from build123d import *

# Parameters (mm, degrees)
SKETCH_R      = 19.5
PAD_DEPTH     = 10
PAD001_START  = 10
SKETCH002_R   = 20
PAD001_DEPTH  = 110
SKETCH003_R   = 18.5
POCKET_DEPTH  = 120.001
PAD003_START  = 118
SKETCH007_R   = 30
SKETCH007_R_2 = 20
PAD003_DEPTH  = 2


with BuildPart() as part:
    # Sketch → Pad (new body)
    with BuildSketch(Plane.XY):
        Circle(SKETCH_R)
    extrude(amount=PAD_DEPTH)

    # Sketch002 → Pad001 (join)
    with BuildSketch(Plane.XY.offset(PAD001_START)):
        Circle(SKETCH002_R)
    extrude(amount=PAD001_DEPTH)

    # Sketch003 → Pocket (cut, through all)
    with BuildSketch(Plane.XY):
        Circle(SKETCH003_R)
    extrude(amount=POCKET_DEPTH, mode=Mode.SUBTRACT)

    # Sketch007 → Pad003 (join)
    with BuildSketch(Plane.XY.offset(PAD003_START)):
        Circle(SKETCH007_R)
        Circle(SKETCH007_R_2, mode=Mode.SUBTRACT)
    extrude(amount=PAD003_DEPTH)


solid = part.part
The model under review builds one solid part; all positions refer to its coordinate system, in mm. A direction names the side the tool comes from. Round coordinates to 2 decimals unless told otherwise and drop trailing zeros. Order: outer loops, then holes, each group sorted by start corner. A loop starts at its lowest first (then second) coordinate and runs counter-clockwise, first axis right, second up. Notation, with made-up numbers: (-39, -28.75) -> (-4, -28.75) arc R11 cw to (-4, -22.75) -> close; hole circle Ø9 at (70, -23.75). An arc over 180 degrees is marked (long way). Write item = value, one per line. Start each with the question number.
Item 1: Clearance check with flat-ended pins moving along their axes: pin 1 Ø6 at (y, z) = (-0.5, 24.5) entering from +X; pin 2 Ø1 at (y, z) = (-4, 33.5) entering from +X; pin 3 Ø1 at (y, z) = (6, 43.5) entering from -X. State where each tip first meets the part, or that it passes through.
Item 2: For faces 1 (the face through (19.2, -4.4, 10)), 2 (the face through (17.24, -7.13, 0)), list the 3-axis set-ups (+Z, -Z, +X, -X, +Y, -Y) from which the entire face can be reached by the end or side of a thin tool; tool diameter is ignored.
Item 3: For line 1 along Y through (x, z) = (0, 66); line 2 along Z through (x, y) = (-19, 7.5); line 3 along Y through (x, z) = (15, 9), list the stretches that pass through material, from the lowest coordinate up.
Item 4: Consider section A-A on x = 0. Write out the cut boundary in (y, z).
Item 5: Consider section C-C on z = 107.5. Write out the cut boundary in (x, y).
Item 6: Consider section D-D on y = -22.5. Write out the cut boundary in (x, z).
Item 7: Mouldability with a two-part tool opening along X and no side actions: class faces 3 (the face through (-4.01, -18.06, 59.16)), 4 (the face through (6, -20, 118)), 5 (the face through (-2.539, 19.334, 4.93)) as released by +X, released by -X, zero draft, split by the parting line, or undercut.
Conclusion:
q1.pin_1 = 20
q1.pin_2 = 19.69
q1.pin_3 = -19.23
q2.face_1 = -Z
q2.face_2 = -Z, +X, -X, +Y, -Y
q3.line_1 = -20 to -18.5, 18.5 to 20
q3.line_2 = 118 to 120
q3.line_3 = -12.46 to -10.83, 10.83 to 12.46
q4.outline = (-30, 118) -> (-20, 118) -> (-20, 10) -> (-19.5, 10) -> (-19.5, 0) -> (-18.5, 0) -> (-18.5, 120) -> (-30, 120) -> close; (18.5, 0) -> (19.5, 0) -> (19.5, 10) -> (20, 10) -> (20, 118) -> (30, 118) -> (30, 120) -> (18.5, 120) -> close
q5.outline = circle Ø40 at (0, 0); hole circle Ø37 at (0, 0)
q6.outline = (-19.84, 118) -> (19.84, 118) -> (19.84, 120) -> (-19.84, 120) -> close
q7.face_3 = undercut
q7.face_4 = zero draft
q7.face_5 = split by the parting line
